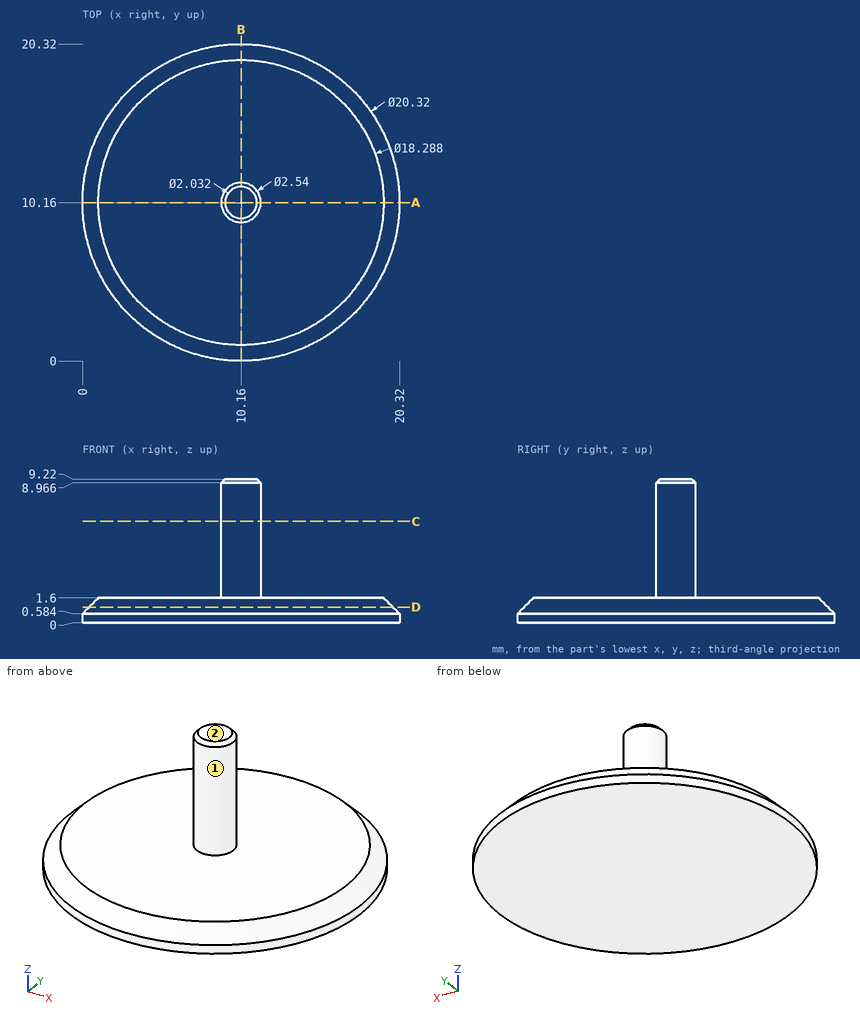
Design review of the part shown in the three views and the two pictorial views. Dimensions are in mm from the part's minimum x, y and z. A direction names the side the tool comes from. Coordinates: 2 decimals unless noted, no trailing zeros. Loops run counter-clockwise (first coordinate to the right, second up) from the corner with the lowest first, then second, coordinate; pieces in that order, holes last. Notation, with made-up numbers: (-27, -16) - (15, -16) arc R16 cw to (15, -4) - close; hole circle Ø9 at (25, 78). An arc over 180 degrees is marked (long way). Use a Markdown table: item, result. Add a question column.
Item 1: We need section A-A (y = 10.16). Give the boundary of the cut face in (x, z), and give its area (3 significant figures).
Item 2: Insertion check: pin 1 Ø4 at (x, y) = (17, 18) entering from -Z; pin 2 Ø3 at (y, z) = (17.5, 5) entering from +X. Each pin has a flat end and moves straight along its axis. Give the tip position at first contact, or say it passes through.
Item 3: We need section C-C (z = 6.5). Give the boundary of the cut face in (x, y).
Item 4: For line 1 (Z direction, x = 4, y = 5.75); line 2 (Z direction, x = 3, y = 4.25); line 3 (X direction, y = 5, z = 0.5), list the stretches that pass through material, from the lowest coordinate up.
Item 5: We need section D-D (z = 1). Give the boundary of the cut face in (x, y), and give its area (3 significant figures).
Item 6: Tool access review of the marked faces 1 and 2: name each direction out of +Z, -Z, +X, -X, +Y, -Y from which nothing blocks a thin tool from reaching the whole face with its end or side.
Results list:
| question | item | result |
|---|---|---|
| 1 | outline | (0, 0) - (20.32, 0) - (20.32, 0.58) - (19.3, 1.6) - (11.43, 1.6) - (11.43, 8.97) - (11.18, 9.22) - (9.14, 9.22) - (8.89, 8.97) - (8.89, 1.6) - (1.02, 1.6) - (0, 0.58) - close |
| 1 | area | 50.8 mm^2 |
| 2 | pin 1 | stops at z = 0 |
| 2 | pin 2 | passes through |
| 3 | outline | circle Ø2.54 at (10.16, 10.16) |
| 4 | line 1 | z = 0 to 1.6 |
| 4 | line 2 | z = 0 to 1.46 |
| 4 | line 3 | x = 1.41 to 18.91 |
| 5 | outline | circle Ø19.49 at (10.16, 10.16) |
| 5 | area | 298 mm^2 |
| 6 | face 1 | +Z |
| 6 | face 2 | +Z, +X, -X, +Y, -Y |
